Work out the finished part from the listing and answer in its coordinate system (mm). Give positions to 0.01 mm unless a question says otherwise; leave off trailing zeros. Write each loop counter-clockwise with the first axis right and the second up, starting at its lowest first coordinate (ties: lowest second). Pieces come first, ordered by that corner, then holes. Notation, with made-up numbers: (81.25, 74.25) - (133.25, 74.25) arc R22 cw to (133.25, 97.25) - close; hole circle Ø10 at (26.25, 62.25). An arc over 180 degrees is marked (long way). Write item = value, one per line.
from build123d import *

# Parameters (mm, degrees)
SKETCH1_W           = 38.1
SKETCH1_H           = 120
BOSS_EXTRUDE1_DEPTH = 38.1
SKETCH2_W           = 34.925
SKETCH2_H           = 34.925
CUT_EXTRUDE1_DEPTH  = 130.767142413
SKETCH18_W          = 3.175
SKETCH18_H          = 3.175
CUT_EXTRUDE3_DEPTH  = 130.767142413
SKETCH19_R          = 3
CUT_EXTRUDE4_DEPTH  = 121.228267267
SKETCH20_W          = 34.925
SKETCH20_H          = 5
CUT_EXTRUDE5_DEPTH  = 121.228267267
SKETCH21_W          = 34.925
SKETCH21_H          = 23.7
CUT_EXTRUDE6_DEPTH  = 121.228267267


with BuildPart() as part:
    # Sketch1 → Boss-Extrude1 (new body)
    with BuildSketch(Plane.XZ.offset(34.925)):
        with Locations((15.875, -55)):
            Rectangle(SKETCH1_W, SKETCH1_H)
    extrude(amount=-BOSS_EXTRUDE1_DEPTH)

    # Sketch2 → Cut-Extrude1 (cut, through all)
    with BuildSketch(Plane(origin=(0, 0, -115), x_dir=(-1, 0, 0), z_dir=(0, 0, -1))):
        with Locations((-17.4625, -17.4625)):
            Rectangle(SKETCH2_W, SKETCH2_H)
    extrude(amount=-CUT_EXTRUDE1_DEPTH, mode=Mode.SUBTRACT)

    # Sketch18 → Cut-Extrude3 (cut, through all)
    with BuildSketch(Plane.XY.offset(5)):
        with Locations((-1.5875, 1.5875)):
            Rectangle(SKETCH18_W, SKETCH18_H)
    extrude(amount=-CUT_EXTRUDE3_DEPTH, mode=Mode.SUBTRACT)


with BuildPart() as body_2:
    # of the pieces the cut leaves, the one that is kept (cut_extrude3_keep)
    add(part.part.solids().sort_by_distance((34.925, 0, -115))[0])

    # Sketch19 → Cut-Extrude4 (cut, through all)
    with BuildSketch(Plane.XZ):
        with Locations(Location((4.7625, -6, 0), (0, 0, 270))):
            Circle(SKETCH19_R)
        with Locations(Location((30.1625, -6, 0), (0, 0, 270))):
            Circle(SKETCH19_R)
        with Locations(Location((17.4625, -83.29, 0), (0, 0, 270))):
            Circle(SKETCH19_R)
        with Locations(Location((17.4625, -25.3, 0), (0, 0, 270))):
            Circle(SKETCH19_R)
    extrude(amount=-CUT_EXTRUDE4_DEPTH, mode=Mode.SUBTRACT)

    # Sketch20 → Cut-Extrude5 (cut, through all)
    with BuildSketch(Plane.XZ):
        with Locations((17.4625, 2.5)):
            Rectangle(SKETCH20_W, SKETCH20_H)
    extrude(amount=-CUT_EXTRUDE5_DEPTH, mode=Mode.SUBTRACT)

    # Sketch21 → Cut-Extrude6 (cut, through all)
    with BuildSketch(Plane.XZ):
        with Locations((17.4625, -103.15)):
            Rectangle(SKETCH21_W, SKETCH21_H)
    extrude(amount=-CUT_EXTRUDE6_DEPTH, mode=Mode.SUBTRACT)


solid = body_2.part
1. For a pull along X with two mould halves and no side action, classify faces 1 (the flat face through (17, 2, -91.3)), 2 (the flat face through (34.925, 2, -46)), 3 (the cylindrical face through (27.234, 1.565, -5.35)) as pulls with the +X half, pulls with the -X half, needs draft (parallel to the pull), parting line crosses it, or undercut.
Solution:
face_1 = needs draft
face_2 = pulls with the +X half
face_3 = undercut
2. Given pin 1 (7 mm diameter, centred on x = 4.76, z = -6, fed in from -Y); pin 2 (5.5 mm diameter, centred on x = 30.16, z = -6, fed in from +Y), each flat-ended and moving along its own axis, determine where each tip first touches the part or whether it passes through.
Solution:
pin_1 = 0
pin_2 = through
3. Find section D-D, the plane y = 0.65. Give the vertices of the cut face in (x, z) (1 decimal).
Solution:
outline = (0, -91.3) - (34.9, -91.3) - (34.9, 0) - (0, 0) - close; hole circle Ø6 at (4.8, -6); hole circle Ø6 at (17.5, -83.3); hole circle Ø6 at (17.5, -25.3); hole circle Ø6 at (30.2, -6)
4. Find section A-A, the plane z = -25.3. Give the vertices of the cut face in (x, y) (1 decimal), then the cut area to 3 significant figures.
Solution:
outline = (0, 0) - (14.5, 0) - (14.5, 3.2) - (0, 3.2) - close; (20.5, 0) - (34.9, 0) - (34.9, 3.2) - (20.5, 3.2) - close
area = 91.8 mm^2
5. Find section B-B, the plane z = -6. Give the vertices of the cut face in (x, y) (1 decimal).
Solution:
outline = (0, 0) - (1.8, 0) - (1.8, 3.2) - (0, 3.2) - close; (7.8, 0) - (27.2, 0) - (27.2, 3.2) - (7.8, 3.2) - close; (33.2, 0) - (34.9, 0) - (34.9, 3.2) - (33.2, 3.2) - close
6. Find section C-C, the plane x = 16. Give the vertices of the cut face in (y, z) (3 decimals), then the cut area to 3 significant figures.
Solution:
outline = (0, -91.3) - (3.175, -91.3) - (3.175, -85.909) - (0, -85.909) - close; (0, -80.671) - (3.175, -80.671) - (3.175, -27.919) - (0, -27.919) - close; (0, -22.681) - (3.175, -22.681) - (3.175, 0) - (0, 0) - close
area = 257 mm^2
7. Straight lines are drawn through the part: line 1 (X direction, y = 2.05, z = -6) (1 decimal); line 2 (X direction, y = 2.35, z = -83.29) (1 decimal); line 3 (Z direction, x = 19, y = 1.6). For each, find the intervals that lie inside material, in ascending order.
Solution:
line_1 = 0 to 1.8, 7.8 to 27.2, 33.2 to 34.9
line_2 = 0 to 14.5, 20.5 to 34.9
line_3 = -91.3 to -85.87, -80.71 to -27.88, -22.72 to 0
